Autodesk Fusion 360 part; units mm, degrees
sketch "Sketch1" plane through (0, 0, 0) normal (0, 0, 1) x (1, 0, 0)
  circle A0 centre (0, 0) radius 43
  line L0 (-3, 5) -> (-3, 38.6919)
  line L1 (-3, 42.9158) -> (3, 42.9158)
  line L2 (3, 38.6608) -> (3, 5)
  line L3 (5, -3) -> (38.6722, -3)
  line L4 (42.8866, -3) -> (42.8866, 3)
  line L5 (38.7134, 3) -> (5, 3)
  line L6 (3, -5) -> (3, -38.6755)
  line L7 (3, -42) -> (-3, -42)
  line L8 (-3, -38.6545) -> (-3, -5)
  line L9 (-5, 3) -> (-38.6589, 3)
  line L10 (-42.9177, 3) -> (-42.9177, -3)
  line L11 (-38.6701, -3) -> (-5, -3)
  arc A1 (3, 5) -> (5, 3) centre (5, 5) ccw
  arc A2 (5, -3) -> (3, -5) centre (5, -5) ccw
  arc A3 (-3, -5) -> (-5, -3) centre (-5, -5) ccw
  arc A4 (-5, 3) -> (-3, 5) centre (-5, 5) ccw
  line L12 (5.2163, 40.649) -> (5.8611, 40.5789)
  arc A5 (5.2163, 40.649) -> (3, 38.6608) centre (5, 38.6608) ccw
  line L13 (-5.1884, 40.683) -> (-4.7244, 40.7269)
  arc A6 (-3, 38.6919) -> (-5.1884, 40.683) centre (-5, 38.6919) ccw
  arc A7 (38.7134, 3) -> (40.7062, 5.169) centre (38.7134, 5) ccw
  line L14 (40.6615, -5.2061) -> (40.6365, -5.4474)
  arc A8 (40.6615, -5.2061) -> (38.6722, -3) centre (38.6722, -5) ccw
  line L15 (5.2032, -40.6651) -> (5.3266, -40.6525)
  arc A9 (3, -38.6755) -> (5.2032, -40.6651) centre (5, -38.6755) ccw
  line L16 (-5.2218, -40.6421) -> (-6.0887, -40.5454)
  arc A10 (-5.2218, -40.6421) -> (-3, -38.6545) centre (-5, -38.6545) ccw
  line L17 (-40.6592, -5.208) -> (-40.6262, -5.5237)
  arc A11 (-38.6701, -3) -> (-40.6592, -5.208) centre (-38.6701, -5) ccw
  line L18 (-40.647, 5.2179) -> (-40.5692, 5.9278)
  arc A12 (-40.647, 5.2179) -> (-38.6589, 3) centre (-38.6589, 5) ccw
  arc A13 (5.3266, -40.6525) -> (40.6365, -5.4474) centre (0, 0) ccw
  arc A14 (-40.6262, -5.5237) -> (-6.0887, -40.5454) centre (0, 0) ccw
  arc A15 (40.7093, 4.8734) -> (5.8611, 40.5789) centre (0, 0) ccw
  arc A16 (-4.7244, 40.7269) -> (-40.5692, 5.9278) centre (0, 0) ccw
  circle A17 centre (0, 0) radius 1.5
  dimension "d1" = 86
  dimension "d2" = 82
  dimension "d7" = 2
  dimension "d8" = 2
  dimension "d9" = 2
  dimension "d10" = 2
  dimension "d11" = 2
  dimension "d12" = 2
  dimension "d13" = 2
  dimension "d14" = 2
  dimension "d15" = 2
  dimension "d16" = 2
  dimension "d17" = 2
  dimension "d18" = 2
  dimension "d19" = 3
extrude "Extrude1" add sketch "Sketch1" along normal blind 3 contours A0 L1 L10
Geometry check sheet. Reference: the model listing, model coordinates, mm. A direction names the side the tool comes from. Round coordinates to 2 decimals unless told otherwise and drop trailing zeros. Order: outer loops, then holes, each group sorted by start corner. A loop starts at its lowest first (then second) coordinate and runs counter-clockwise, first axis right, second up. Notation, with made-up numbers: M -1.75,1 L 19.25,1 A21 cw 19.25,14 Z; hole C -23,47 d3. An arc over 180 degrees is marked long. Write each question's results on one line, items separated by ' | '. Start each with the question number.
1. Cross-section at B-B on x = 0. Record the boundary of the cut face in (y, z), plus the area to 3 significant figures.
2. Go/stop test with flat-tipped pins: P1, Ø1.5, axis at x = 23.5, z = 1.5, coming from the +Y side; P2, Ø0.9, axis at x = 18.5, z = 2, coming from the -Y side; P3, Ø1.5, axis at x = -19, z = 1.5, coming from the -Y side. Record where each tip stops, or that it passes through.
3. Cross-section at C-C on y = 14.5. Record the boundary of the cut face in (x, z).
4. Material ranges on L1, parallel to Y at x = 0, z = 2.2; L2, parallel to X at y = 6, z = 0.6; L3, parallel to X at y = -24, z = 0.5, recorded low to high. Write a range as from..to.
5. Set-up check for faces 3 (the face through (-42.918, 0, 1)), 4 (the face through (29.21, -28.77, 1.48)): record each of +Z, -Z, +X, -X, +Y, -Y from which the full face is reachable in a straight line by a thin tool's end or side.
6. Draft check along X on faces 1 (the face through (-30.72, 30.09, 1.48)), 2 (the face through (-3.61, 40.13, 1.48)). Enter one of: pulls with the +X half, pulls with the -X half, needs draft (parallel to the pull), parting line crosses it, or undercut.
7. Cross-section at D-D on x = -13. Record the boundary of the cut face in (y, z), plus the area to 3 significant figures.
8. Cross-section at A-A on y = 0. Record the boundary of the cut face in (x, z).
Resolved:
1) outline: M -43,0 L -1.5,0 L -1.5,3 L -43,3 Z; M 1.5,0 L 42.92,0 L 42.92,3 L 1.5,3 Z | area: 249 mm2
2) P1: y = 36.49 | P2: y = -39.03 | P3: y = -38.94
3) outline: M -40.48,0 L -38.35,0 L -38.35,3 L -40.48,3 Z; M -3,0 L 3,0 L 3,3 L -3,3 Z; M 38.35,0 L 40.48,0 L 40.48,3 L 38.35,3 Z
4) L1: -43..-1.5, 1.5..42.92 | L2: -42.58..-40.56, -3..3, 40.56..42.58 | L3: -35.68..-33.24, -3..3, 33.24..35.68
5) face 3: +Z, -Z, -X, +Y, -Y | face 4: +Z, -Z
6) face 1: pulls with the -X half | face 2: undercut
7) outline: M -40.99,0 L -38.88,0 L -38.88,3 L -40.99,3 Z; M -3,0 L 3,0 L 3,3 L -3,3 Z; M 38.88,0 L 40.99,0 L 40.99,3 L 38.88,3 Z | area: 30.6 mm2
8) outline: M -42.92,0 L -1.5,0 L -1.5,3 L -42.92,3 Z; M 1.5,0 L 43,0 L 43,3 L 1.5,3 Z
